```python
from build123d import *

# Parameters (mm, degrees)
SKETCH1_W           = 330.2
SKETCH1_H           = 139.7
BOSS_EXTRUDE1_DEPTH = 1.5748
SKETCH6_R           = 25
CUT_EXTRUDE3_DEPTH  = 180.27496338
CUT_EXTRUDE4_DEPTH  = 4


with BuildPart() as part:
    # Sketch1 → Boss-Extrude1 (new body)
    with BuildSketch(Plane.XY):
        Rectangle(SKETCH1_W, SKETCH1_H)
    extrude(amount=BOSS_EXTRUDE1_DEPTH)

    # Sketch6 → Cut-Extrude3 (cut, through all)
    with BuildSketch(Plane.XY.offset(1.5748)):
        with Locations((108.75, 0)):
            Circle(SKETCH6_R)
        with Locations((7.861, 0)):
            Circle(SKETCH6_R)
        with Locations((-92.774, 0)):
            Circle(SKETCH6_R)
    extrude(amount=-CUT_EXTRUDE3_DEPTH, mode=Mode.SUBTRACT)

    # Sketch8 → Cut-Extrude4 (cut)
    with BuildSketch(Plane.XY.offset(1.5748)):
        with BuildLine():
            Line((88.120489669, -22.53869864), (86.21130136, -20.629510331))
            ThreePointArc((86.21130136, -20.629510331), (85.625514922, -19.215296769), (86.21130136, -17.801083206))
            Line((86.21130136, -17.801083206), (88.862951789, -15.149432777))
            ThreePointArc((88.862951789, -15.149432777), (91.07233047, -17.67766953), (93.600567223, -19.887048211))
            Line((93.600567223, -19.887048211), (90.948916794, -22.53869864))
            ThreePointArc((90.948916794, -22.53869864), (89.534703231, -23.124485078), (88.120489669, -22.53869864))
        make_face()
        with BuildLine():
            Line((131.28869864, 17.801083206), (128.637048211, 15.149432777))
            ThreePointArc((128.637048211, 15.149432777), (126.42766953, 17.67766953), (123.899432777, 19.887048211))
            Line((123.899432777, 19.887048211), (126.551083206, 22.53869864))
            ThreePointArc((126.551083206, 22.53869864), (127.965296769, 23.124485078), (129.379510331, 22.53869864))
            Line((129.379510331, 22.53869864), (131.28869864, 20.629510331))
            ThreePointArc((131.28869864, 20.629510331), (131.874485078, 19.215296769), (131.28869864, 17.801083206))
        make_face()
        with BuildLine():
            Line((30.39969864, 17.801083206), (27.748048211, 15.149432777))
            ThreePointArc((27.748048211, 15.149432777), (25.53866953, 17.67766953), (23.010432777, 19.887048211))
            Line((23.010432777, 19.887048211), (25.662083206, 22.53869864))
            ThreePointArc((25.662083206, 22.53869864), (27.076296769, 23.124485078), (28.490510331, 22.53869864))
            Line((28.490510331, 22.53869864), (30.39969864, 20.629510331))
            ThreePointArc((30.39969864, 20.629510331), (30.985485078, 19.215296769), (30.39969864, 17.801083206))
        make_face()
        with BuildLine():
            Line((-7.288432777, -19.887048211), (-9.940083206, -22.53869864))
            ThreePointArc((-9.940083206, -22.53869864), (-11.354296769, -23.124485078), (-12.768510331, -22.53869864))
            Line((-12.768510331, -22.53869864), (-14.67769864, -20.629510331))
            ThreePointArc((-14.67769864, -20.629510331), (-15.263485078, -19.215296769), (-14.67769864, -17.801083206))
            Line((-14.67769864, -17.801083206), (-12.026048211, -15.149432777))
            ThreePointArc((-12.026048211, -15.149432777), (-9.81666953, -17.67766953), (-7.288432777, -19.887048211))
        make_face()
        with BuildLine():
            Line((-115.31269864, -17.801083206), (-112.661048211, -15.149432777))
            ThreePointArc((-112.661048211, -15.149432777), (-110.45166953, -17.67766953), (-107.923432777, -19.887048211))
            Line((-107.923432777, -19.887048211), (-110.575083206, -22.53869864))
            ThreePointArc((-110.575083206, -22.53869864), (-111.989296769, -23.124485078), (-113.403510331, -22.53869864))
            Line((-113.403510331, -22.53869864), (-115.31269864, -20.629510331))
            ThreePointArc((-115.31269864, -20.629510331), (-115.898485078, -19.215296769), (-115.31269864, -17.801083206))
        make_face()
        with BuildLine():
            Line((-70.23530136, 17.801083206), (-72.886951789, 15.149432777))
            ThreePointArc((-72.886951789, 15.149432777), (-75.09633047, 17.67766953), (-77.624567223, 19.887048211))
            Line((-77.624567223, 19.887048211), (-74.972916794, 22.53869864))
            ThreePointArc((-74.972916794, 22.53869864), (-73.558703231, 23.124485078), (-72.144489669, 22.53869864))
            Line((-72.144489669, 22.53869864), (-70.23530136, 20.629510331))
            ThreePointArc((-70.23530136, 20.629510331), (-69.649514922, 19.215296769), (-70.23530136, 17.801083206))
        make_face()
    extrude(amount=-CUT_EXTRUDE4_DEPTH, mode=Mode.SUBTRACT)


solid = part.part
```
Work out the finished part from the listing and answer in its coordinate system (mm). Give positions to 0.01 mm unless a question says otherwise; leave off trailing zeros. Loops run counter-clockwise (first coordinate to the right, second up) from the corner with the lowest first, then second, coordinate; pieces in that order, holes last. Notation, with made-up numbers: (-38, -36.5) - (-29, -36.5) arc R17 cw to (-29, -6.5) - close; hole circle Ø7 at (56.5, 3). An arc over 180 degrees is marked (long way). Use CSV: the item, a comma, the result in double quotes. Start each with the question number.
(1) Find section B-B, the plane x = 104.5. Determine the outline of the cut face in (y, z), plus the area to 3 significant figures.
(2) Find the intervals of material crossed by L1, parallel to X at y = 3.5, z = 0.6; L2, parallel to X at y = -10, z = 1.2; L3, parallel to Y at x = -75.5, z = 1.2, in increasing order.
(3) Find section D-D, the plane x = -94.5. Determine the outline of the cut face in (y, z).
(4) Find section A-A, the plane y = 11. Determine the outline of the cut face in (x, z), plus the area to 3 significant figures.
(5) Determine the mould class of faces 1 (the face through (-2, 32, 1.575)), 2 (the face through (-110.09, 18.03, 0.8)) for opening direction X: released by +X, released by -X, zero draft, split by the parting line, or undercut.
(6) Find section C-C, the plane z = 0.5. Count the separate pieces of the cut face and the enclosed holes in it, plus the area to 3 significant figures.
Results found:
1,outline,"(-69.85, 0) - (-24.64, 0) - (-24.64, 1.57) - (-69.85, 1.57) - close; (24.64, 0) - (69.85, 0) - (69.85, 1.57) - (24.64, 1.57) - close"
1,area,"142 mm^2"
2,L1,"-165.1 to -117.53, -68.02 to -16.89, 32.61 to 84, 133.5 to 165.1"
2,L2,"-165.1 to -115.69, -69.86 to -15.05, 30.77 to 85.84, 131.66 to 165.1"
2,L3,"-69.85 to -18.07, 22.01 to 69.85"
3,outline,"(-69.85, 0) - (-24.94, 0) - (-24.94, 1.57) - (-69.85, 1.57) - close; (24.94, 0) - (69.85, 0) - (69.85, 1.57) - (24.94, 1.57) - close"
4,outline,"(-165.1, 0) - (-115.22, 0) - (-115.22, 1.57) - (-165.1, 1.57) - close; (-70.32, 0) - (-14.59, 0) - (-14.59, 1.57) - (-70.32, 1.57) - close; (30.31, 0) - (86.3, 0) - (86.3, 1.57) - (30.31, 1.57) - close; (131.2, 0) - (165.1, 0) - (165.1, 1.57) - (131.2, 1.57) - close"
4,area,"308 mm^2"
5,face 1,"zero draft"
5,face 2,"undercut"
6,separate pieces,"1"
6,enclosed holes,"3"
6,area,"40,000 mm^2"
